Source: CAD feature listing. Evaluate the final solid. Frame: model axes, mm. Face numbers are marked on the shaded views. A direction names the side the tool comes from. Coordinates: 2 decimals unless noted, no trailing zeros. Order: outer loops, then holes, each group sorted by start corner. A loop starts at its lowest first (then second) coordinate and runs counter-clockwise, first axis right, second up.
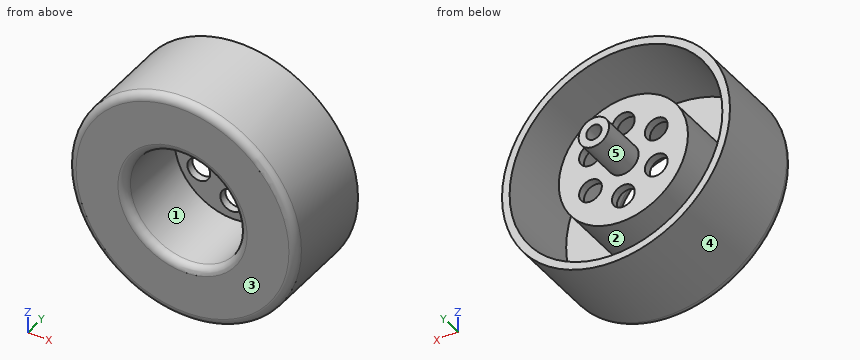
```python
from build123d import *

# Parameters (mm, degrees)
F0_R      = 19.05
F1_DEPTH  = 7.9375
F2_R      = 9.525
F3_DEPTH  = 12.7
F4_T      = -1.27
F5_R      = 1.905
F6_DEPTH  = 3.176
F7_R      = 2.54
F8_DEPTH  = 7.62
F9_R      = 1.27
F10_DEPTH = 21.591
F11_R     = 1.27


with BuildPart() as f1:
    # F0 (on Front) → F1 (new body, symmetric)
    with BuildSketch(Plane.XZ):
        Circle(F0_R)
    extrude(amount=F1_DEPTH, both=True)

    # F2 (on face) → F3 (cut)
    with BuildSketch(Plane.XZ.offset(7.9375)):
        Circle(F2_R)
    extrude(amount=-F3_DEPTH, mode=Mode.SUBTRACT)

    # F4
    f4_openings = [f1.faces().sort_by_distance(p)[0] for p in [
        (0, 7.9375, 0),
    ]]
    offset(amount=F4_T, openings=f4_openings, kind=Kind.INTERSECTION)

    # F5 (on face) → F6 (cut, through all)
    with BuildSketch(Plane.XZ.offset(-4.7625)):
        with Locations((0, 6.35)):
            Circle(F5_R)
        with Locations((-5.499261314, 3.175)):
            Circle(F5_R)
        with Locations((-5.499261314, -3.175)):
            Circle(F5_R)
        with Locations((0, -6.35)):
            Circle(F5_R)
        with Locations((5.499261314, -3.175)):
            Circle(F5_R)
        with Locations((5.499261314, 3.175)):
            Circle(F5_R)
    extrude(amount=-F6_DEPTH, mode=Mode.SUBTRACT)

    # F7 (on face) → F8 (join)
    with BuildSketch(Plane(origin=(0, 6.0325, 0), x_dir=(-1, 0, 0), z_dir=(0, 1, 0))):
        Circle(F7_R)
    extrude(amount=F8_DEPTH)

    # F9 (on face) → F10 (cut, through all)
    with BuildSketch(Plane(origin=(0, 13.6525, 0), x_dir=(-1, 0, 0), z_dir=(0, 1, 0))):
        Circle(F9_R)
    extrude(amount=-F10_DEPTH, mode=Mode.SUBTRACT)

    # F11
    f11_edges = [f1.edges().sort_by_distance(p)[0] for p in [
        (-19.05, -7.9375, 0),
        (-9.525, -7.9375, 0),
    ]]
    fillet(f11_edges, radius=F11_R)


solid = f1.part
```
1. Section query D-D on x = 0. Count the separate pieces of the cut face and the enclosed holes in it, plus the area to 3 significant figures.
Findings:
separate pieces: 4
enclosed holes: 0
area: 123 mm2
2. Pin query (flat end, axial travel): P1, Ø1.5, axis at y = -5, z = 3, coming from the +X side; P2, Ø1.5, axis at x = 1, z = -5, coming from the +Y side; P3, Ø3.5, axis at x = 0, z = -6.35, coming from the -Y side; P4, Ø5, axis at x = 5.5, z = -3.18, coming from the -Y side. Return the tip coordinate at first contact, or that it passes through.
Findings:
P1: stops at x = 18.92
P2: stops at y = 6.03
P3: passes through
P4: stops at y = 4.76
3. Section query B-B on y = -0.5. Return loops of the section in (x, z) (3 decimals), plus the area to 3 significant figures.
Findings:
outline: circle Ø38.1 at (0, 0); circle Ø21.59 at (0, 0); hole circle Ø35.56 at (0, 0); hole circle Ø19.05 at (0, 0)
area: 228 mm2
4. Access query for the marked faces 1 and 2. Directions: +Z, -Z, +X, -X, +Y, -Y. A direction counts if a zero-diameter tool reaches every point of the face in a straight line with its end or side. Return the directions, or none.
Findings:
face 1: -Y
face 2: +Y
5. Section query C-C on y = 8.75. Return loops of the section in (x, z), plus the area to 3 significant figures.
Findings:
outline: circle Ø5.08 at (0, 0); hole circle Ø2.54 at (0, 0)
area: 15.2 mm2
6. Draft query along Z for the marked faces 3, 4 and 5. Return one class per face: released by +Z, released by -Z, zero draft, split by the parting line, or undercut.
Findings:
face 3: zero draft
face 4: split by the parting line
face 5: undercut
7. Ray query, line 1 (X direction, y = -5.25, z = -8); line 2 (X direction, y = 0.5, z = 7.5); line 3 (Z direction, x = -8, y = 5.5). Return the intervals inside material, ascending.
Findings:
line 1: x = -17.29 to -15.88, -7.25 to -5.17, 5.17 to 7.25, 15.88 to 17.29
line 2: x = -17.51 to -16.12, -7.76 to -5.87, 5.87 to 7.76, 16.12 to 17.51
line 3: z = -17.29 to -15.88, -7.25 to 7.25, 15.88 to 17.29
